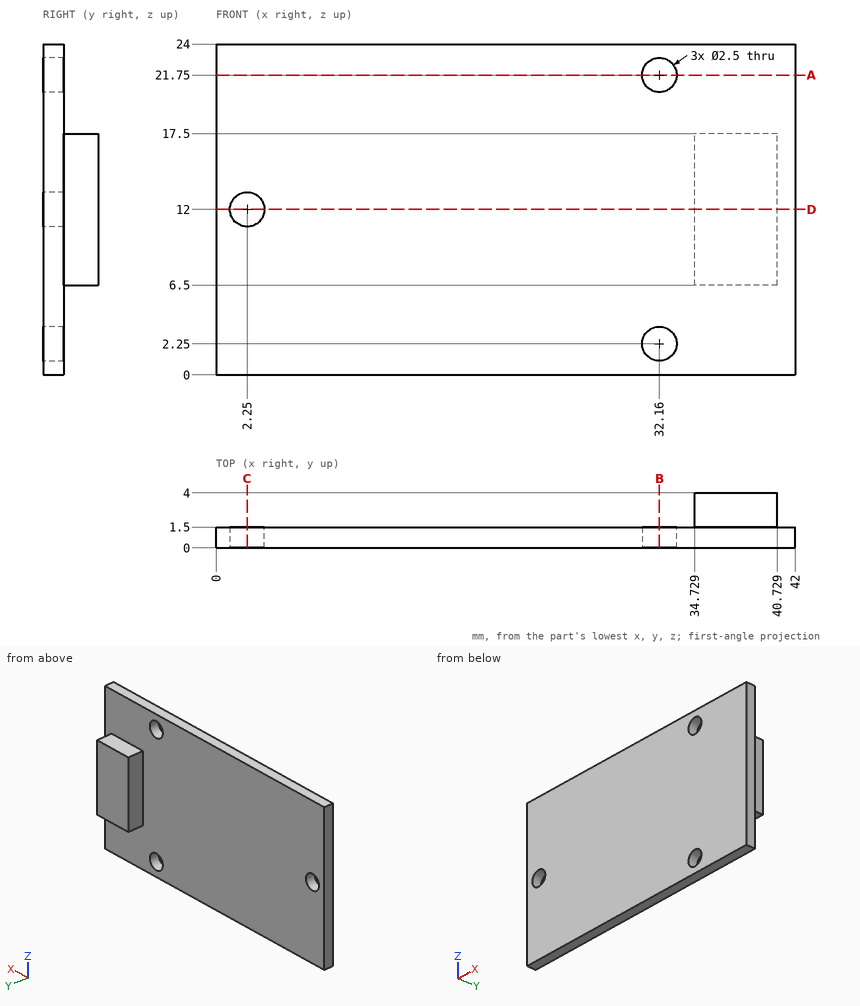
The figure shows three views and two pictorial views of one solid part (mm, origin at its lowest corner). Answer the questions. Coordinates: 2 decimals unless noted, no trailing zeros. Loops run counter-clockwise (first coordinate to the right, second up) from the corner with the lowest first, then second, coordinate; pieces in that order, holes last.
(1) The part is cut by section D-D (z = 12). Determine the outline of the cut face in (x, y).
Solution:
outline: (0, 0) - (1, 0) - (1, 1.5) - (0, 1.5) - close; (3.5, 0) - (42, 0) - (42, 1.5) - (40.73, 1.5) - (40.73, 4) - (34.73, 4) - (34.73, 1.5) - (3.5, 1.5) - close
(2) The part is cut by section A-A (z = 21.75). Determine the outline of the cut face in (x, y).
Solution:
outline: (0, 0) - (30.91, 0) - (30.91, 1.5) - (0, 1.5) - close; (33.41, 0) - (42, 0) - (42, 1.5) - (33.41, 1.5) - close
(3) The part is cut by section B-B (x = 32.16). Determine the outline of the cut face in (y, z), and give its area (3 significant figures).
Solution:
outline: (0, 0) - (1.5, 0) - (1.5, 1) - (0, 1) - close; (0, 3.5) - (1.5, 3.5) - (1.5, 20.5) - (0, 20.5) - close; (0, 23) - (1.5, 23) - (1.5, 24) - (0, 24) - close
area: 28.5 mm2
(4) A flat-ended cylindrical pin translates along its axis: pin 1 Ø5 at (x, z) = (17, 10.5) entering from +Y. Find the tip coordinate at first contact, or state that the pin passes through.
Solution:
pin 1: stops at y = 1.5
(5) Consider line 1 along Z through (x, y) = (32.16, 0.3); line 2 along Z through (x, y) = (2.25, 1.1); line 3 along X through (y, z) = (1.05, 12). Determine where each line is inside the solid, lowest interval first.
Solution:
line 1: z = 0 to 1, 3.5 to 20.5, 23 to 24
line 2: z = 0 to 10.75, 13.25 to 24
line 3: x = 0 to 1, 3.5 to 42
(6) The part is cut by section C-C (x = 2.25). Determine the outline of the cut face in (y, z).
Solution:
outline: (0, 0) - (1.5, 0) - (1.5, 10.75) - (0, 10.75) - close; (0, 13.25) - (1.5, 13.25) - (1.5, 24) - (0, 24) - close
